```python
from build123d import *

# Parameters (mm, degrees)
SKETCH1_W           = 250
SKETCH1_H           = 65
BOSS_EXTRUDE1_DEPTH = 6
SKETCH2_W           = 5.5
SKETCH2_H           = 34
SKETCH2_H_2         = 47.5
CUT_EXTRUDE1_DEPTH  = 259.381500886
SKETCH3_W           = 60
SKETCH3_H           = 21
CUT_EXTRUDE2_DEPTH  = 259.381500886
SKETCH4_W           = 55.5
SKETCH4_H           = 6
CUT_EXTRUDE3_DEPTH  = 259.381500886
SKETCH5_W           = 5.5
SKETCH5_H           = 6.2
BOSS_EXTRUDE2_DEPTH = 6


with BuildPart() as part:
    # Sketch1 → Boss-Extrude1 (new body)
    with BuildSketch(Plane(origin=(0, 0, 0), x_dir=(1, 0, 0), z_dir=(0, 1, 0))):
        with Locations((125, 32.5)):
            Rectangle(SKETCH1_W, SKETCH1_H)
    extrude(amount=BOSS_EXTRUDE1_DEPTH)

    # Sketch2 → Cut-Extrude1 (cut, through all)
    with BuildSketch(Plane(origin=(0, 6, 0), x_dir=(1, 0, 0), z_dir=(0, 1, 0))):
        with Locations((20.75, 38)):
            Rectangle(SKETCH2_W, SKETCH2_H)
        with Locations((50.75, 21)):
            Rectangle(SKETCH2_W, SKETCH2_H_2)
        with Locations((199.25, 21)):
            Rectangle(SKETCH2_W, SKETCH2_H_2)
        with Locations((229.25, 38)):
            Rectangle(SKETCH2_W, SKETCH2_H)
    extrude(amount=-CUT_EXTRUDE1_DEPTH, mode=Mode.SUBTRACT)

    # Sketch3 → Cut-Extrude2 (cut, through all)
    with BuildSketch(Plane(origin=(0, 6, 0), x_dir=(1, 0, 0), z_dir=(0, 1, 0))):
        with Locations((126.5, 10.5)):
            Rectangle(SKETCH3_W, SKETCH3_H)
    extrude(amount=-CUT_EXTRUDE2_DEPTH, mode=Mode.SUBTRACT)

    # Sketch4 → Cut-Extrude3 (cut, through all)
    with BuildSketch(Plane(origin=(0, 6, 0), x_dir=(1, 0, 0), z_dir=(0, 1, 0))):
        with Locations((35.75, 30)):
            Rectangle(SKETCH4_W, SKETCH4_H)
    extrude(amount=-CUT_EXTRUDE3_DEPTH, mode=Mode.SUBTRACT)

    # Sketch5 → Boss-Extrude2 (add)
    with BuildSketch(Plane(origin=(0, 6, 0), x_dir=(1, 0, 0), z_dir=(0, 1, 0))):
        with Locations((50.75, 11.9)):
            Rectangle(SKETCH5_W, SKETCH5_H)
    extrude(amount=-BOSS_EXTRUDE2_DEPTH)


solid = part.part
```
The listing builds one solid part. Answer for the finished solid, in the listing's coordinates (mm). A direction names the side the tool comes from. Give positions to 0.01 mm unless a question says otherwise; leave off trailing zeros. Order: outer loops, then holes, each group sorted by start corner. A loop starts at its lowest first (then second) coordinate and runs counter-clockwise, first axis right, second up. Notation, with made-up numbers: (-12.75, -16.75) -> (42.25, -16.75) arc R26 ccw to (42.25, 2.25) -> close; hole circle Ø7 at (46.25, 49.5). An arc over 180 degrees is marked (long way). Answer as a JSON object with one key per item and string values. Group by question number.
Item 1: The part is cut by section C-C on y = 2.4. Give the number of separate pieces and of enclosed holes in the cut face, and give its area (3 significant figures).
Item 2: Consider L1, parallel to X at y = 4.6, z = -48; L2, parallel to X at y = 5, z = -16; L3, parallel to X at y = 4.3, z = -32.5. Determine where each line is inside the solid, lowest interval first. Write a range as from..to.
Item 3: The part is cut by section A-A on z = -4. Write down the section's boundary in (x, y), and give its area (3 significant figures).
Item 4: The part is cut by section B-B on z = -37. Write down the section's boundary in (x, y), and give its area (3 significant figures).
Item 5: Flat-ended cylindrical pins translate along their axes: pin 1 (3 mm diameter, centred on x = 82.5, y = 4, fed in from +Z); pin 2 (1.5 mm diameter, centred on x = 51.5, y = 3.5, fed in from +Z). Find the tip coordinate at first contact, or state that the pin passes through.
Item 6: Determine the mould class of faces 1 (the flat face through (229, 3, -55)), 2 (the flat face through (176, 3, 0)), 3 (the flat face through (196.5, 3, -22)) for opening direction X: pulls with the +X half, pulls with the -X half, needs draft (parallel to the pull), parting line crosses it, or undercut.
Item 7: A tool of negligible diameter and unlimited length cuts with its end or side. For faces 4 (the flat face through (199, 3, -44.75)), 5 (the flat face through (229, 3, -21)), 6 (the flat face through (24, 3, 0)), from which of +Z, -Z, +X, -X, +Y, -Y can it reach the whole face along a straight path? Write none if from no direction.
Item 8: The part is cut by section D-D on x = 120. Write down the section's boundary in (y, z).
Result set:
{
 "1": {"separate pieces": "1", "enclosed holes": "2", "area": "13,900 mm²"},
 "2": {"L1": "0..18, 23.5..226.5, 232..250", "L2": "0..48, 53.5..96.5, 156.5..196.5, 202..250", "L3": "0..8, 63.5..196.5, 202..226.5, 232..250"},
 "3": {"outline": "(0, 0) -> (48, 0) -> (48, 6) -> (0, 6) -> close; (53.5, 0) -> (96.5, 0) -> (96.5, 6) -> (53.5, 6) -> close; (156.5, 0) -> (196.5, 0) -> (196.5, 6) -> (156.5, 6) -> close; (202, 0) -> (250, 0) -> (250, 6) -> (202, 6) -> close", "area": "1,070 mm²"},
 "4": {"outline": "(0, 0) -> (18, 0) -> (18, 6) -> (0, 6) -> close; (23.5, 0) -> (48, 0) -> (48, 6) -> (23.5, 6) -> close; (53.5, 0) -> (196.5, 0) -> (196.5, 6) -> (53.5, 6) -> close; (202, 0) -> (226.5, 0) -> (226.5, 6) -> (202, 6) -> close; (232, 0) -> (250, 0) -> (250, 6) -> (232, 6) -> close", "area": "1,370 mm²"},
 "5": {"pin 1": "z = 0", "pin 2": "z = -8.8"},
 "6": {"face 1": "undercut", "face 2": "needs draft", "face 3": "undercut"},
 "7": {"face 4": "+Z, +Y, -Y", "face 5": "+Y, -Y", "face 6": "+Z, +X, -X, +Y, -Y"},
 "8": {"outline": "(0, -65) -> (6, -65) -> (6, -21) -> (0, -21) -> close"}
}
